The listing builds one solid part. Answer for the finished solid, in the listing's coordinates (mm). A direction names the side the tool comes from. Round coordinates to 2 decimals unless told otherwise and drop trailing zeros. Write each loop counter-clockwise with the first axis right and the second up, starting at its lowest first coordinate (ties: lowest second). Pieces come first, ordered by that corner, then holes. Notation, with made-up numbers: (-33.75, 24.5) - (22.25, 24.5) arc R15 cw to (22.25, 33.5) - close; hole circle Ø8 at (47.5, 6). An arc over 180 degrees is marked (long way). Use a Markdown table: item, result. Add a question column.
1) A cutting plane is placed at C-C (x = -154). Give the vertices of the cut face in (y, z) (3 decimals).
2) This flat-tipped pin is pushed along its axis until it touches: P1, Ø11, axis at x = 71.5, z = 0, coming from the +Y side. Where does it stop, or does it pass through?
3) A tool of negligible diameter and unlimited length cuts with its end or side. For faces 1 (the flat face through (5, 0.534, -1)), 2 (the cylindrical face through (155.642, -1.88, 0.209)), from which of +Z, -Z, +X, -X, +Y, -Y can it reach the whole face along a straight path? Write none if from no direction.
4) Find the intervals of material crossed by probe 1 along Z at (x, y) = (100, 3.75) (3 decimals); probe 2 along Z at (x, y) = (204.85, -3.2); probe 3 along Y at (x, z) = (-14, -9), in increasing order. Write a range as from..to.
5) A cutting plane is placed at B-B (y = 5). Give the vertices of the cut face in (x, z) (3 decimals).
6) Determine the mould class of faces 3 (the cylindrical face through (101.3, -1.88, -1.82)), 4 (the flat face through (5, -4.228, -1)), 5 (the flat face through (-195.2, 0, -1)) for opening direction X: +X half, -X half, draft (parallel to the pull), parting line (faces both ways), or undercut.
```python
from build123d import *

# Parameters (mm, degrees)
BOSS_EXTRUDE1_DEPTH = 16
SCALE1_SCALE        = 25.4
SKETCH2_R           = 4.7625
CUT_EXTRUDE1_DEPTH  = 12.112499989


with BuildPart() as part:
    # Sketch1 → Boss-Extrude1 (new body)
    with BuildSketch(Plane(origin=(0, 0, 0), x_dir=(0, 0, -1), z_dir=(1, 0, 0))):
        Polygon((0, 0.4375), (0, 0), (1.75, 0), (1.75, 0.4375), (1.375, 0.4375), (1.375, 0.1875), (0.375, 0.1875), (0.375, 0.4375), align=None)
    extrude(amount=BOSS_EXTRUDE1_DEPTH)


with BuildPart() as part_1:
    # Scale1: scaled about (8, 0.173295455, -0.875)
    add(part.part.scale(SCALE1_SCALE).moved(Location((-195.2, -4.228409102, 21.35))))

    # Sketch2 → Cut-Extrude1 (cut, through all)
    with BuildSketch(Plane.XZ.offset(4.228409091)):
        with Locations((-176.15, 0)):
            Circle(SKETCH2_R)
        with Locations((-163.45, 0)):
            Circle(SKETCH2_R)
        with Locations((-128.525, 0)):
            Circle(SKETCH2_R)
        with Locations((-64.23125, 0)):
            Circle(SKETCH2_R)
        with Locations((71.5, 0)):
            Circle(SKETCH2_R)
        with Locations((96.9, 0)):
            Circle(SKETCH2_R)
        with Locations((135, 0)):
            Circle(SKETCH2_R)
        with Locations((160.4, 0)):
            Circle(SKETCH2_R)
        with Locations((204.85, 0)):
            Circle(SKETCH2_R)
    extrude(amount=-CUT_EXTRUDE1_DEPTH, mode=Mode.SUBTRACT)


solid = part_1.part
```
Entries:
| question | item | result |
|---|---|---|
| 1 | outline | (-4.228, -23.1) - (6.884, -23.1) - (6.884, -13.575) - (0.534, -13.575) - (0.534, 11.825) - (6.884, 11.825) - (6.884, 21.35) - (-4.228, 21.35) - close |
| 2 | P1 | stops at y = 0.53 |
| 3 | face 1 | +X, -X, +Y |
| 3 | face 2 | +Y, -Y |
| 4 | probe 1 | z = -23.1..-13.575, 11.825..21.35 |
| 4 | probe 2 | z = -23.1..-4.76, 4.76..21.35 |
| 4 | probe 3 | y = -4.23..0.53 |
| 5 | outline | (-195.2, -23.1) - (211.2, -23.1) - (211.2, -13.575) - (-195.2, -13.575) - close; (-195.2, 11.825) - (211.2, 11.825) - (211.2, 21.35) - (-195.2, 21.35) - close |
| 6 | face 3 | undercut |
| 6 | face 4 | draft |
| 6 | face 5 | -X half |
